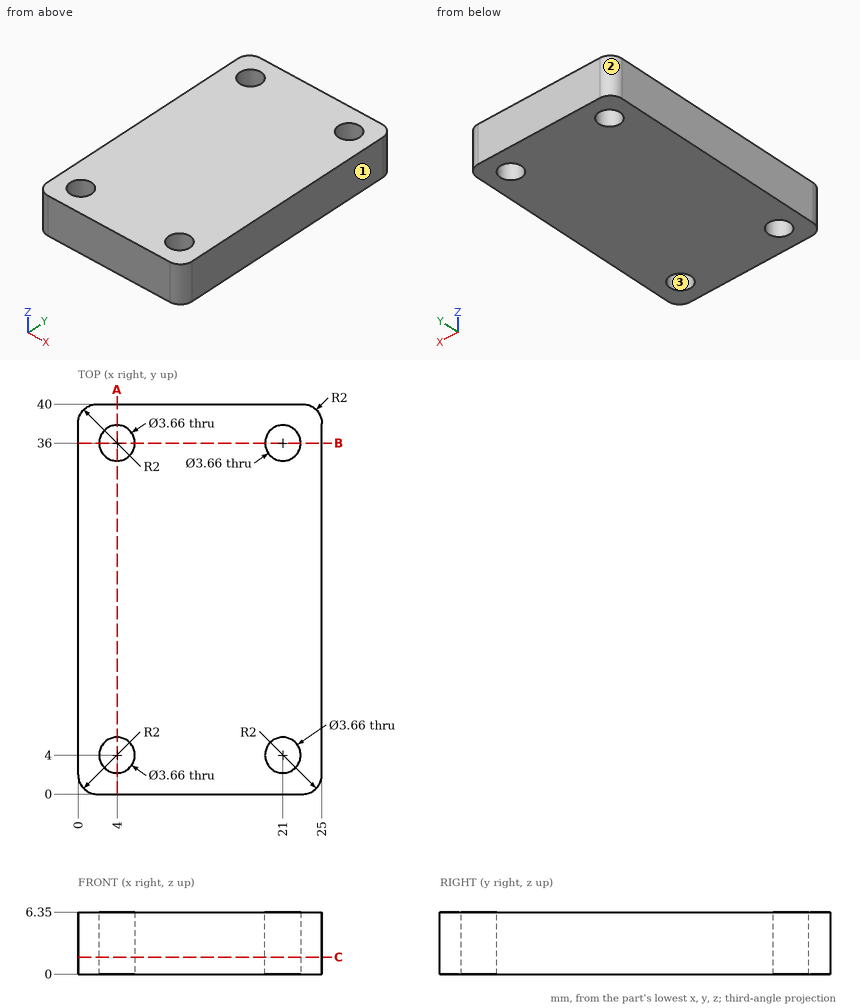
Verification items for this drawing (mm, ordinates from the low corner). Coordinates: 2 decimals unless noted, no trailing zeros. Write each loop counter-clockwise with the first axis right and the second up, starting at its lowest first coordinate (ties: lowest second). Pieces come first, ordered by that corner, then holes. Notation, with made-up numbers: (74, 34.5) -> (125, 34.5) arc R35 ccw to (125, 71.5) -> close; hole circle Ø2 at (67, 36). An arc over 180 degrees is marked (long way). One line per item, written item: value. Start each with the question number.
Q1. Cross-section at A-A on x = 4. Enter the section's corners in (y, z), and give its area (3 significant figures).
Q2. Cross-section at B-B on y = 36. Enter the section's corners in (x, z), and give its area (3 significant figures).
Q3. Cross-section at C-C on z = 1.75. Enter the section's corners in (x, y).
Q4. Mould release check, pull along Y, two halves, no side actions. Record for the marked faces 1, 2 and 3: pulls with the +Y half, pulls with the -Y half, needs draft (parallel to the pull), parting line crosses it, or undercut.
Q5. Thickness scan on L1, parallel to Y at x = 21, z = 5; L2, parallel to Y at x = 5, z = 3; L3, parallel to X at y = 3, z = 3.5. Record the ranges inside material, lowest first. Write a range as from..to.
Q6. Go/stop test with flat-tipped pins: P1, Ø1, axis at x = 6.5, y = 27.5, coming from the -Z side; P2, Ø3.5, axis at x = 4, y = 4, coming from the +Z side. Record where each tip stops, or that it passes through.
Checked values:
1. outline: (0, 0) -> (2.17, 0) -> (2.17, 6.35) -> (0, 6.35) -> close; (5.83, 0) -> (34.17, 0) -> (34.17, 6.35) -> (5.83, 6.35) -> close; (37.83, 0) -> (40, 0) -> (40, 6.35) -> (37.83, 6.35) -> close
1. area: 208 mm²
2. outline: (0, 0) -> (2.17, 0) -> (2.17, 6.35) -> (0, 6.35) -> close; (5.83, 0) -> (19.17, 0) -> (19.17, 6.35) -> (5.83, 6.35) -> close; (22.83, 0) -> (25, 0) -> (25, 6.35) -> (22.83, 6.35) -> close
2. area: 112 mm²
3. outline: (0, 2) arc R2 ccw to (2, 0) -> (23, 0) arc R2 ccw to (25, 2) -> (25, 38) arc R2 ccw to (23, 40) -> (2, 40) arc R2 ccw to (0, 38) -> close; hole circle Ø3.66 at (4, 4); hole circle Ø3.66 at (4, 36); hole circle Ø3.66 at (21, 4); hole circle Ø3.66 at (21, 36)
4. face 1: needs draft
4. face 2: pulls with the +Y half
4. face 3: undercut
5. L1: y = 0..2.17, 5.83..34.17, 37.83..40
5. L2: y = 0..2.47, 5.53..34.47, 37.53..40
5. L3: x = 0..2.47, 5.53..19.47, 22.53..25
6. P1: stops at z = 0
6. P2: passes through
